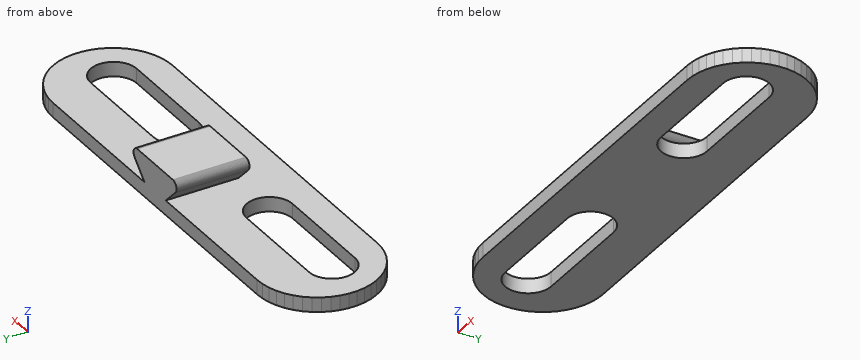
from build123d import *

# Parameters (mm, degrees)
BOSS_EXTRUDE1_DEPTH = 1.39999995
CUT_EXTRUDE1_DEPTH  = 2.39999995
BOSS_EXTRUDE2_DEPTH = 6.99999975


with BuildPart() as part:
    # Sketch1 → Boss-Extrude1 (new body)
    with BuildSketch(Plane.XY.offset(-1.200000057)):
        Polygon((17.170472071, 2.74639437), (16.38751477, 2.799950074), (-16.38751477, 2.799950074), (-17.170472071, 2.74639437), (-17.93884486, 2.586724702), (-18.678320572, 2.323914785), (-19.375121221, 1.962861512), (-20.016269758, 1.510289963), (-20.589821041, 0.974630471), (-21.085090935, 0.365861692), (-21.492853761, -0.304676127), (-21.80551365, -1.024491969), (-22.017247975, -1.780177932), (-22.12410979, -2.557656262), (-22.12410979, -3.342443844), (-22.017247975, -4.119921941), (-21.80551365, -4.875607789), (-21.492853761, -5.595424213), (-21.085090935, -6.265962031), (-20.589821041, -6.874730811), (-20.016269758, -7.410389837), (-19.375121221, -7.862961851), (-18.678320572, -8.224015124), (-17.93884486, -8.48682411), (-17.170472071, -8.646493778), (-16.38751477, -8.700050414), (16.38751477, -8.700050414), (17.170472071, -8.646493778), (17.93884486, -8.48682411), (18.678320572, -8.224015124), (19.375121221, -7.862961851), (20.016269758, -7.410389837), (20.589821041, -6.874730811), (21.085090935, -6.265962031), (21.492853761, -5.595424213), (21.80551365, -4.875607789), (22.017247975, -4.119921941), (22.12410979, -3.342443844), (22.12410979, -2.557656262), (22.017247975, -1.780177932), (21.80551365, -1.024491969), (21.492853761, -0.304676127), (21.085090935, 0.365861692), (20.589821041, 0.974630471), (20.016269758, 1.510289963), (19.375121221, 1.962861512), (18.678320572, 2.323914785), (17.93884486, 2.586724702), align=None)
    extrude(amount=-BOSS_EXTRUDE1_DEPTH)

    # Sketch2 → Cut-Extrude1 (cut, through all)
    with BuildSketch(Plane.XY.offset(-1.200000057)):
        with BuildLine():
            Line((-7.499999832, -5.900050048), (-17.500000075, -5.900050048))
            ThreePointArc((-17.500000075, -5.900050048), (-19.700000075, -3.700050048), (-17.500000075, -1.500050048))
            Line((-17.500000075, -1.500050048), (-7.499999832, -1.500050048))
            ThreePointArc((-7.499999832, -1.500050048), (-5.299999832, -3.700050048), (-7.499999832, -5.900050048))
        make_face()
    cut_extrude1 = extrude(amount=-CUT_EXTRUDE1_DEPTH, mode=Mode.SUBTRACT)

    # Mirror1: Cut-Extrude1 across plane
    add(cut_extrude1.mirror(Plane(origin=(0, 0, 0), x_dir=(0, 0, 1), z_dir=(1, 0, 0))), mode=Mode.SUBTRACT)

    # Sketch4 → Boss-Extrude2 (add)
    with BuildSketch(Plane(origin=(0, 2.799950074, 0), x_dir=(1, 0, 0), z_dir=(0, 1, 0))):
        Polygon((3.330282168, -0.438419171), (3.275736002, -0.375735923), (1.700000023, 1.200000057), (-1.700000023, 1.200000057), (-3.275736002, -0.375735923), (-3.330282168, -0.438419171), (-3.375645261, -0.508037279), (-3.410955193, -0.583254965), (-3.435534658, -0.662629609), (-3.448912408, -0.744638965), (-3.450831631, -0.827709911), (-3.441255772, -0.910249539), (-3.420368303, -0.990674831), (-3.388569923, -1.067443052), (-3.346470417, -1.139081782), (-3.294877242, -1.204217318), (-3.234779928, -1.261600293), (-3.167331219, -1.310130116), (-3.093824489, -1.348876162), (-3.015669761, -1.377095236), (-2.934365766, -1.394246239), (-2.851471771, -1.39999995), (2.851471771, -1.39999995), (2.934365766, -1.394246239), (3.015669761, -1.377095236), (3.093824489, -1.348876162), (3.167331219, -1.310130116), (3.234779928, -1.261600293), (3.294877242, -1.204217318), (3.346470417, -1.139081782), (3.388569923, -1.067443052), (3.420368303, -0.990674831), (3.441255772, -0.910249539), (3.450831631, -0.827709911), (3.448912408, -0.744638965), (3.435534658, -0.662629609), (3.410955193, -0.583254965), (3.375645261, -0.508037279), align=None)
    extrude(amount=-BOSS_EXTRUDE2_DEPTH)


solid = part.part
Here's how the part is built. I have some questions about the finished solid (model axes, mm). Round coordinates to 2 decimals unless told otherwise and drop trailing zeros. Order: outer loops, then holes, each group sorted by start corner. A loop starts at its lowest first (then second) coordinate and runs counter-clockwise, first axis right, second up. Notation, with made-up numbers: (-40, 72) -> (19, 72) arc R12 ccw to (19, 76) -> close; hole circle Ø9 at (20.25, -6.75). An arc over 180 degrees is marked (long way). Return JSON: item names as keys, results as strings.
Q1. If we section it at A-A on z = -0.35: List the corners of the cut face in (x, y) for me, plus the area to 3 significant figures.
Filled sheet:
{"outline": "(-2.55, -4.2) -> (2.55, -4.2) -> (2.55, 2.8) -> (-2.55, 2.8) -> close", "area": "35.7 mm^2"}
Q2. I need wall thicknesses on line 1 along X through (y, z) = (-5.5, -2.4); line 2 along X through (y, z) = (-3, -1.6); line 3 along Z through (x, y) = (0.5, -5.75). Which ranges of each line are inside material? Lowest first, please. Write a range as from..to.
Filled sheet:
{"line 1": "x = -21.53..-18.76, -6.24..6.24, 18.76..21.53", "line 2": "x = -22.12..-19.59, -5.41..5.41, 19.59..22.12", "line 3": "z = -2.6..-1.2"}
Q3. For pin 1 Ø2 at (x, z) = (4, 0) entering from -Y; pin 2 Ø2 at (y, z) = (-1, -0.5) entering from +X, each with a flat end and sliding along its axis, tell me the tip position at first contact or that it passes through.
Filled sheet:
{"pin 1": "stops at y = -4.2", "pin 2": "stops at x = 22"}
